Check sheet for the modelled part. Datum: model origin and axes. Units: mm. A direction names the side the tool comes from. Give positions to 0.01 mm unless a question says otherwise; leave off trailing zeros. Order: outer loops, then holes, each group sorted by start corner. A loop starts at its lowest first (then second) coordinate and runs counter-clockwise, first axis right, second up. Notation, with made-up numbers: (-21, 63.5) -> (38, 63.5) arc R10 cw to (38, 82.5) -> close; hole circle Ø6 at (-8.75, -13). An arc over 180 degrees is marked (long way). Answer in a Markdown table with one row per item. Add a question column.
(1) Thickness scan on L1, parallel to Y at x = -50, z = 20.5; L2, parallel to X at y = -20.5, z = 20; L3, parallel to Y at x = -51, z = 18.5. Record the ranges inside material, lowest first. Write a range as [from, to].
(2) Go/stop test with flat-tipped pins: pin 1 (4.5 mm diameter, centred on x = -49.49, y = -92.53, fed in from +Z); pin 2 (8 mm diameter, centred on y = -95.5, z = 15.5, fed in from +X); pin 3 (6.5 mm diameter, centred on y = -18, z = 21.5, fed in from -X); pin 4 (5 mm diameter, centred on x = 21.51, y = -21.53, fed in from +Z). Record where each tip stops, or that it passes through.
(3) Cross-section at A-A (y = -52.5). Record the cut outline in (x, z).
(4) Cross-section at C-C (x = -7.5). Record the cut outline in (y, z), then the cut area to 3 significant figures.
(5) Set-up check for faces 5 (the face through (-3.901, -87.053, 17.643)), 6 (the face through (-39, -10.776, 16)), 7 (the face through (-51.21, -89.37, 16.27)): record each of +Z, -Z, +X, -X, +Y, -Y from which the full face is reachable in a straight line by a thin tool's end or side.
(6) Cross-section at D-D (y = -16). Record the cut outline in (x, z).
(7) Release check for a two-part mould opening along X. For faces 1 (the face through (-61, -66.018, 16)), 2 (the face through (10.104, -103.203, 16.269)), 3 (the face through (-9.491, -22, 16)), 4 (the face through (22.72, -19.63, 16.27)) record: released by +X, released by -X, zero draft, split by the parting line, or undercut.
(8) Cross-section at B-B (z = 17.5). Record the cut outline in (x, y), then the cut area to 3 significant figures.
```python
from build123d import *

# Parameters (mm, degrees)
SKETCH1_R           = 2.25
SKETCH1_R_2         = 2.372088477
BOSS_EXTRUDE1_DEPTH = 33
SKETCH2_R           = 29.45
CUT_EXTRUDE1_DEPTH  = 31.15
SKETCH3_W           = 29.3
SKETCH3_H           = 53.492504466
CUT_EXTRUDE2_DEPTH  = 58


with BuildPart() as part:
    # Sketch1 → Boss-Extrude1 (new body)
    with BuildSketch(Plane.XY):
        with BuildLine():
            Line((-67.490537214, -8.925660295), (-67.490537214, -66.018164761))
            Line((-67.490537214, -66.018164761), (-55.315435977, -66.018164761))
            ThreePointArc((-55.315435977, -66.018164761), (-52.985618491, -76.806821645), (-48.344940443, -86.82117505))
            Line((-48.344940443, -86.82117505), (-54.153009969, -91.989482541))
            ThreePointArc((-54.153009969, -91.989482541), (-52.996606833, -95.645534427), (-49.499657733, -97.218852767))
            Line((-49.499657733, -97.218852767), (-43.732472201, -92.086925876))
            ThreePointArc((-43.732472201, -92.086925876), (-23.877416965, -105.274546325), (-0.103624015, -106.99015709))
            ThreePointArc((-0.103624015, -106.99015709), (10.241918426, -103.132381102), (19.415070822, -96.986979642))
            ThreePointArc((19.415070822, -96.986979642), (34.927027694, -62.122719509), (21.114082576, -26.551101781))
            Line((21.114082576, -26.551101781), (25.392497534, -22.761995578))
            ThreePointArc((25.392497534, -22.761995578), (24.56016132, -18.82386048), (20.751489025, -17.521667342))
            Line((20.751489025, -17.521667342), (16.336215646, -21.431979902))
            ThreePointArc((16.336215646, -21.431979902), (0.541775721, -12.152351096), (-17.490537214, -8.925660295))
            Line((-17.490537214, -8.925660295), (-67.490537214, -8.925660295))
        make_face()
        with Locations((21.509462786, -21.525660295)):
            Circle(SKETCH1_R, mode=Mode.SUBTRACT)
        with Locations((-49.490537214, -92.525660295)):
            Circle(SKETCH1_R_2, mode=Mode.SUBTRACT)
    extrude(amount=BOSS_EXTRUDE1_DEPTH)

    # Sketch2 → Cut-Extrude1 (cut)
    with BuildSketch(Plane.XY.offset(33)):
        with Locations((-17.490537214, -60.925660295)):
            Circle(SKETCH2_R)
    extrude(amount=-CUT_EXTRUDE1_DEPTH, mode=Mode.SUBTRACT)

    # Sketch3 → Cut-Extrude2 (cut)
    with BuildSketch(Plane.ZY.offset(67.490537214)):
        with Locations((16.5, -37.521912528)):
            Rectangle(SKETCH3_W, SKETCH3_H)
    extrude(amount=-CUT_EXTRUDE2_DEPTH, mode=Mode.SUBTRACT)


solid = part.part
```
Answer below:
| question | item | result |
|---|---|---|
| 1 | L1 | y = [-97.19, -94.84], [-90.21, -88.29], [-83.87, -64.27], [-10.78, -8.93] |
| 1 | L2 | x = [-9.49, 15.22], [17.39, 19.51], [23.51, 25.45] |
| 1 | L3 | y = [-96.97, -94.36], [-90.7, -89.18], [-81.82, -64.27], [-10.78, -8.93] |
| 2 | pin 1 | passes through |
| 2 | pin 2 | stops at x = 24.41 |
| 2 | pin 3 | stops at x = -9.49 |
| 2 | pin 4 | stops at z = 33 |
| 3 | outline | (-67.49, 0) -> (34.22, 0) -> (34.22, 33) -> (10.73, 33) -> (10.73, 1.85) -> (-67.49, 1.85) -> close; (-67.49, 31.15) -> (-45.71, 31.15) -> (-45.71, 33) -> (-67.49, 33) -> close |
| 4 | outline | (-107.77, 0) -> (-9.89, 0) -> (-9.89, 33) -> (-33.22, 33) -> (-33.22, 1.85) -> (-88.63, 1.85) -> (-88.63, 33) -> (-107.77, 33) -> close |
| 4 | area | 1,500 mm² |
| 5 | face 5 | +Z |
| 5 | face 6 | -X |
| 5 | face 7 | +Z, -Z, -X |
| 6 | outline | (-67.49, 0) -> (8.7, 0) -> (8.7, 33) -> (-67.49, 33) -> (-67.49, 31.15) -> (-9.49, 31.15) -> (-9.49, 1.85) -> (-67.49, 1.85) -> close |
| 7 | face 1 | zero draft |
| 7 | face 2 | released by +X |
| 7 | face 3 | released by -X |
| 7 | face 4 | undercut |
| 8 | outline | (-67.49, -66.02) -> (-55.32, -66.02) arc R49.99 ccw to (-48.34, -86.82) -> (-54.15, -91.99) arc R4.69 ccw to (-49.5, -97.22) -> (-43.73, -92.09) arc R46.86 ccw to (-0.1, -106.99) arc R47.43 ccw to (19.42, -96.99) arc R49.64 ccw to (21.11, -26.55) -> (25.39, -22.76) arc R4.08 ccw to (20.75, -17.52) -> (16.34, -21.43) arc R52 ccw to (-17.49, -8.93) -> (-67.49, -8.93) -> (-67.49, -10.78) -> (-9.49, -10.78) -> (-9.49, -32.58) arc R29.45 cw (long way) to (-46.75, -64.27) -> (-67.49, -64.27) -> close; hole circle Ø4.74 at (-49.49, -92.53); hole circle Ø4.5 at (21.51, -21.53) |
| 8 | area | 3,420 mm² |
